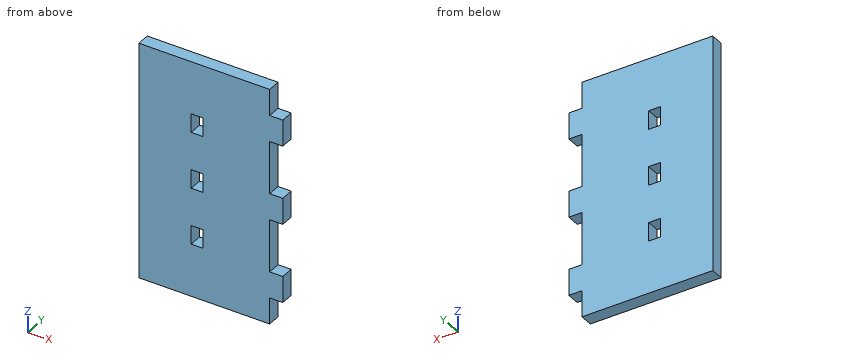
Autodesk Inventor part; units mm, degrees
ref_plane "YZ Plane" through (0, 0, 0) normal (1, 0, 0) x (0, 1, 0)
ref_plane "XZ Plane" through (0, 0, 0) normal (0, 1, 0) x (-1, 0, 0)
ref_plane "XY Plane" through (0, 0, 0) normal (0, 0, 1) x (1, 0, 0)
sketch "Sketch1" plane through (0, 0, 0) normal (0, 1, 0) x (-1, 0, 0)
  line L0 (0, 0) -> (63.5, 0)
  line L1 (63.5, 0) -> (63.5, -114.3)
  line L2 (63.5, -114.3) -> (0, -114.3)
  line L3 (0, -114.3) -> (0, 0)
  line L4 (38.1, -52.6288) -> (32.4358, -52.6288)
  line L5 (32.4358, -52.6288) -> (32.4358, -61.6712)
  line L6 (32.4358, -61.6712) -> (38.1, -61.6712)
  line L7 (38.1, -61.6712) -> (38.1, -52.6288)
  line L8 (38.1, -25.4) -> (32.4358, -25.4)
  line L9 (32.4358, -25.4) -> (32.4358, -34.4424)
  line L10 (32.4358, -34.4424) -> (38.1, -34.4424)
  line L11 (38.1, -34.4424) -> (38.1, -25.4)
  line L12 (38.1, -79.8576) -> (32.4358, -79.8576)
  line L13 (32.4358, -79.8576) -> (32.4358, -88.9)
  line L14 (32.4358, -88.9) -> (38.1, -88.9)
  line L15 (38.1, -88.9) -> (38.1, -79.8576)
  dimension "d0" = 63.5
  dimension "d1" = 114.3
  dimension "d2" = 5.6642
  dimension "d3" = 9.0424
  dimension "d4" = 5.6642
  dimension "d5" = 9.0424
  dimension "d8" = 5.6642
  dimension "d9" = 9.0424
  dimension "d10" = 25.4
  dimension "d11" = 25.4
  dimension "d12" = 25.4
  dimension "d13" = 25.4
  dimension "d14" = 25.4
  dimension "d15" = 45.4152
  dimension "d16" = 18.1864
  dimension "d17" = 18.1864
extrude "Extrusion1" add sketch "Sketch1" along normal blind 6.35
sketch "Sketch2" plane through (0, 0, 0) normal (0, -1, 0) x (1, 0, 0)
  line L0 (0, -101.6) -> (6.35, -101.6)
  line L1 (6.35, -101.6) -> (6.35, -88.9)
  line L2 (6.35, -88.9) -> (0, -88.9)
  line L3 (0, -88.9) -> (0, -101.6)
  line L4 (-63.5, -114.3) -> (0, -114.3)
  line L5 (0, 0) -> (0, -114.3)
  line L6 (0, -25.4) -> (6.35, -25.4)
  line L7 (6.35, -25.4) -> (6.35, -12.7)
  line L8 (6.35, -12.7) -> (0, -12.7)
  line L9 (0, -12.7) -> (0, -25.4)
  line L10 (0, -63.5) -> (6.35, -63.5)
  line L11 (6.35, -63.5) -> (6.35, -50.8)
  line L12 (6.35, -50.8) -> (0, -50.8)
  line L13 (0, -50.8) -> (0, -63.5)
  dimension "d20" = 6.35
  dimension "d21" = 12.7
  dimension "d22" = 12.7
  dimension "d23" = 6.35
  dimension "d24" = 12.7
  dimension "d25" = 12.7
  dimension "d26" = 6.35
  dimension "d27" = 12.7
  dimension "d28" = 63.5
  dimension "d29" = 25.4
extrude "Extrusion2" add sketch "Sketch2" against normal blind 6.35
equation "\"d11\" = d10"
equation "\"d12\" = d11"
properties part number "LEDFront"
Source: CAD feature listing. Evaluate the final solid. Frame: model axes, mm. Give positions to 0.01 mm unless a question says otherwise; leave off trailing zeros. Loops run counter-clockwise (first coordinate to the right, second up) from the corner with the lowest first, then second, coordinate; pieces in that order, holes last. Notation, with made-up numbers: (35.5, 48) - (57.5, 48) arc R24 ccw to (57.5, 72) - close; hole circle Ø3 at (-25.5, 51.5). An arc over 180 degrees is marked (long way). Use CSV: the item, a comma, the result in double quotes. Start each with the question number.
1. Pin query (flat end, axial travel): pin 1 (3 mm diameter, centred on y = 4.5, z = -107, fed in from +X); pin 2 (1.9 mm diameter, centred on x = 4.5, y = 3, fed in from +Z); pin 3 (3 mm diameter, centred on x = 2.5, y = 4.5, fed in from -Z). Return the tip coordinate at first contact, or that it passes through.
2. Section B-B (y = 4.5). Output: boundary loops of the cut face in (x, z), then the cut area to 3 significant figures.
3. Section A-A (z = -31). Output: boundary loops of the cut face in (x, y).
4. Section C-C (z = -67). Output: boundary loops of the cut face in (x, y).
5. Ray query, L1, parallel to Z at x = -36.5, y = 4.5; L2, parallel to X at y = 0.5, z = -28.5; L3, parallel to X at y = 5, z = -60.5. Return the intervals inside material, ascending.
Response:
1,pin 1,"x = 0"
1,pin 2,"z = -12.7"
1,pin 3,"z = -101.6"
2,outline,"(-63.5, -114.3) - (0, -114.3) - (0, -101.6) - (6.35, -101.6) - (6.35, -88.9) - (0, -88.9) - (0, -63.5) - (6.35, -63.5) - (6.35, -50.8) - (0, -50.8) - (0, -25.4) - (6.35, -25.4) - (6.35, -12.7) - (0, -12.7) - (0, 0) - (-63.5, 0) - close; hole (-38.1, -88.9) - (-32.44, -88.9) - (-32.44, -79.86) - (-38.1, -79.86) - close; hole (-38.1, -61.67) - (-32.44, -61.67) - (-32.44, -52.63) - (-38.1, -52.63) - close; hole (-38.1, -34.44) - (-32.44, -34.44) - (-32.44, -25.4) - (-38.1, -25.4) - close"
2,area,"7,350 mm²"
3,outline,"(-63.5, 0) - (-38.1, 0) - (-38.1, 6.35) - (-63.5, 6.35) - close; (-32.44, 0) - (0, 0) - (0, 6.35) - (-32.44, 6.35) - close"
4,outline,"(-63.5, 0) - (0, 0) - (0, 6.35) - (-63.5, 6.35) - close"
5,L1,"-114.3 to -88.9, -79.86 to -61.67, -52.63 to -34.44, -25.4 to 0"
5,L2,"-63.5 to -38.1, -32.44 to 0"
5,L3,"-63.5 to -38.1, -32.44 to 6.35"
